Could you check a few things on this model? Use its own coordinates, in mm. A direction names the side the tool comes from. Round coordinates to 2 decimals unless told otherwise and drop trailing zeros. Loops run counter-clockwise (first coordinate to the right, second up) from the corner with the lowest first, then second, coordinate; pieces in that order, holes last. Notation, with made-up numbers: (58.5, -24.5) -> (103.5, -24.5) arc R25 cw to (103.5, 5.5) -> close; hole circle Ø2 at (21.25, -10). An arc over 180 degrees is marked (long way). Put each result on its own line as item: value. Start each with the question number.
1. Imagine slicing it at B-B, the plane z = 0. Please give me the cut outline in (x, y), and give its area (3 significant figures).
2. If we mould it in two halves opening along Z, with no side actions, what happens to faces 3 (the cylindrical face through (-35.876, 0.986, -7.967)), 4 (the flat face through (-16, 0, -1)), 5 (the flat face through (7, 1, -24))? For each: pulls with the +Z half, pulls with the -Z half, needs draft (parallel to the pull), parting line crosses it, or undercut.
3. Imagine slicing it at A-A, the plane x = 0. Please give me the cut outline in (y, z), and give its area (3 significant figures).
4. I need wall thicknesses on line 1 (X direction, y = 1.35, z = 0); line 2 (Z direction, x = 3, y = 0.5); line 3 (Z direction, x = -6.5, y = 1.7). Which ranges of each line are inside material? Lowest first, please. Write a range as [from, to].
5. Which directions (+Z, -Z, +X, -X, +Y, -Y) give clear straight access to the entire face, cutting with the end or side of a thin tool? Please do faces 1 (the flat face through (0, 1, -16.864)), 2 (the flat face through (-16, 2, -1)).
6. Imagine slicing it at C-C, the plane y = 1.15. Please give me the cut outline in (x, z), and give its area (3 significant figures).
7. Imagine slicing it at D-D, the plane x = 20.5. Please give me the cut outline in (y, z), and give its area (3 significant figures).
8. I'm going to push flat-ended pins straight in: P1, Ø0.6, axis at y = 1.5, z = -27.5, coming from the -X side; P2, Ø0.6, axis at y = 1, z = 27, coming from the -X side; P3, Ø1, axis at y = 1.5, z = 0, coming from the +X side. Where does each tip first touch, or does it pass through?
```python
from build123d import *

# Parameters (mm, degrees)
SKETCH3_R           = 36.75
BOSS_EXTRUDE1_DEPTH = 2
SKETCH4_R           = 12.5
CUT_EXTRUDE1_DEPTH  = 53.010816183
CUT_EXTRUDE2_DEPTH  = 53.010816183
SKETCH6_W           = 14
SKETCH6_H           = 14
CUT_EXTRUDE3_DEPTH  = 53.010816183
CUT_EXTRUDE4_DEPTH  = 53.010816183


with BuildPart() as part:
    # Sketch3 → Boss-Extrude1 (new body)
    with BuildSketch(Plane(origin=(0, 0, 0), x_dir=(1, 0, 0), z_dir=(0, 1, 0))):
        with Locations(Location((0, 0, 0), (0, 0, 270))):
            Circle(SKETCH3_R)
    extrude(amount=BOSS_EXTRUDE1_DEPTH)

    # Sketch4 → Cut-Extrude1 (cut, through all)
    with BuildSketch(Plane(origin=(0, 0, 0), x_dir=(1, 0, 0), z_dir=(0, 1, 0))):
        with Locations(Location((0, 0, 0), (0, 0, 270))):
            Circle(SKETCH4_R)
    extrude(amount=CUT_EXTRUDE1_DEPTH, mode=Mode.SUBTRACT)

    # Sketch5 → Cut-Extrude2 (cut, through all)
    with BuildSketch(Plane(origin=(0, 2, 0), x_dir=(1, 0, 0), z_dir=(0, 1, 0))):
        Polygon((-30.663619776, 7), (-30.663619776, 0), (-30.663619776, -7), (-16.663619776, -7), (-16.663619776, 7), align=None)
    extrude(amount=-CUT_EXTRUDE2_DEPTH, mode=Mode.SUBTRACT)

    # Sketch6 → Cut-Extrude3 (cut, through all)
    with BuildSketch(Plane(origin=(0, 2, 0), x_dir=(1, 0, 0), z_dir=(0, 1, 0))):
        with Locations((23.218077959, 0)):
            Rectangle(SKETCH6_W, SKETCH6_H)
    extrude(amount=-CUT_EXTRUDE3_DEPTH, mode=Mode.SUBTRACT)

    # Sketch8 → Cut-Extrude4 (cut, through all)
    with BuildSketch(Plane(origin=(0, 0, 0), x_dir=(1, 0, 0), z_dir=(0, 1, 0))):
        Polygon((0, 30.868072457), (-7, 30.868072457), (-7, 16.864385373), (6.999997959, 16.864385373), (6.999997959, 30.868072457), align=None)
        Polygon((0, -31.010274177), (7, -31.010274177), (7, -17.010274177), (-7, -17.010274177), (-7, -31.010274177), align=None)
    extrude(amount=CUT_EXTRUDE4_DEPTH, mode=Mode.SUBTRACT)


solid = part.part
```
Entries:
1. outline: (-36.75, 0) -> (-30.66, 0) -> (-30.66, 2) -> (-36.75, 2) -> close; (-16.66, 0) -> (-12.5, 0) -> (-12.5, 2) -> (-16.66, 2) -> close; (12.5, 0) -> (16.22, 0) -> (16.22, 2) -> (12.5, 2) -> close; (30.22, 0) -> (36.75, 0) -> (36.75, 2) -> (30.22, 2) -> close
1. area: 41.0 mm^2
2. face 3: parting line crosses it
2. face 4: needs draft
2. face 5: undercut
3. outline: (0, -36.75) -> (2, -36.75) -> (2, -30.87) -> (0, -30.87) -> close; (0, -16.86) -> (2, -16.86) -> (2, -12.5) -> (0, -12.5) -> close; (0, 12.5) -> (2, 12.5) -> (2, 17.01) -> (0, 17.01) -> close; (0, 31.01) -> (2, 31.01) -> (2, 36.75) -> (0, 36.75) -> close
3. area: 41.0 mm^2
4. line 1: [-36.75, -30.66], [-16.66, -12.5], [12.5, 16.22], [30.22, 36.75]
4. line 2: [-36.63, -30.87], [-16.86, -12.13], [12.13, 17.01], [31.01, 36.63]
4. line 3: [-36.17, -30.87], [-16.86, -10.68], [10.68, 17.01], [31.01, 36.17]
5. face 1: +Y, -Y
5. face 2: +Z, -Z, +X, -X, +Y
6. outline: circle Ø73.5 at (0, 0); hole (-30.66, -7) -> (-16.66, -7) -> (-16.66, 7) -> (-30.66, 7) -> close; hole circle Ø25 at (0, 0); hole (-7, -30.87) -> (7, -30.87) -> (7, -16.86) -> (-7, -16.86) -> close; hole (-7, 17.01) -> (7, 17.01) -> (7, 31.01) -> (-7, 31.01) -> close; hole (16.22, -7) -> (30.22, -7) -> (30.22, 7) -> (16.22, 7) -> close
6. area: 2,970 mm^2
7. outline: (0, -30.5) -> (2, -30.5) -> (2, -7) -> (0, -7) -> close; (0, 7) -> (2, 7) -> (2, 30.5) -> (0, 30.5) -> close
7. area: 94.0 mm^2
8. P1: x = -24.71
8. P2: x = -25.25
8. P3: x = 36.75
